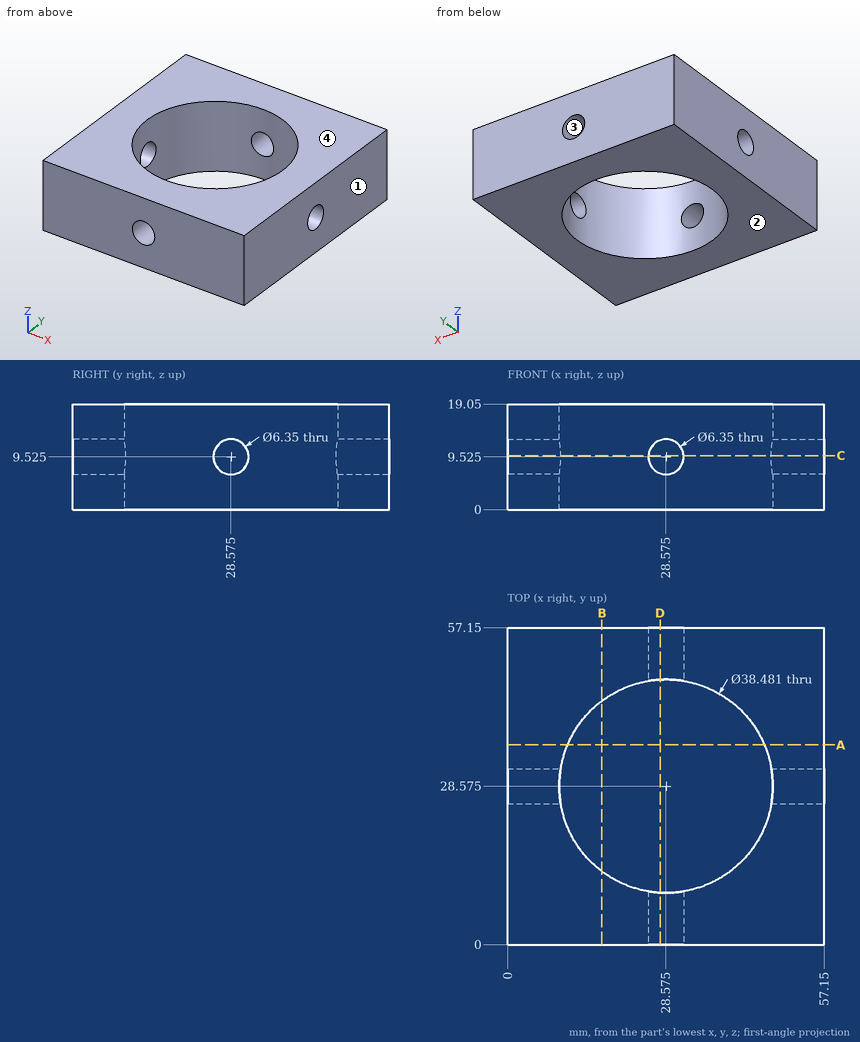
Could you check a few things on this drawing? It's one solid part, dimensions in mm from its lowest x, y, z. Give positions to 0.01 mm unless a question says otherwise; leave off trailing zeros. Loops run counter-clockwise (first coordinate to the right, second up) from the corner with the lowest first, then second, coordinate; pieces in that order, holes last. Notation, with made-up numbers: M -17.75,14 L 9.25,14 A26 cw 9.25,34 Z; hole C 63,35.5 d7. An arc over 180 degrees is marked long. Answer as a JSON object with one key per item and string values.
Q1. If we mould it in two halves opening along Z, with no side actions, what happens to the marked faces 1, 2, 3 and 4? For each: pulls with the +Z half, pulls with the -Z half, needs draft (parallel to the pull), parting line crosses it, or undercut.
Values found:
{"face 1": "needs draft", "face 2": "pulls with the -Z half", "face 3": "undercut", "face 4": "pulls with the +Z half"}
Q2. Suppose I cut it at D-D, the plane x = 27.5. List the corners of the cut face in (y, z) for me, plus the area to 3 significant figures.
Values found:
{"outline": "M 0,0 L 9.36,0 L 9.36,6.54 L 0,6.54 Z; M 0,12.51 L 9.36,12.51 L 9.36,19.05 L 0,19.05 Z; M 47.79,0 L 57.15,0 L 57.15,6.54 L 47.79,6.54 Z; M 47.79,12.51 L 57.15,12.51 L 57.15,19.05 L 47.79,19.05 Z", "area": "245 mm²"}
Q3. Suppose I cut it at C-C, the plane z = 9.75. State how many separate pieces and enclosed holes the cut face has, plus the area to 3 significant figures.
Values found:
{"separate pieces": "4", "enclosed holes": "0", "area": "1,860 mm²"}
Q4. If I drill on probe 1 along X at (y, z) = (5, 9.5); probe 2 along Y at (x, z) = (28, 16.5); probe 3 along X at (y, z) = (11, 15.25), over which ranges is the centre line in solid material (lowest first)? Write a range as [from, to].
Values found:
{"probe 1": "x = [0, 25.4], [31.75, 57.15]", "probe 2": "y = [0, 9.34], [47.81, 57.15]", "probe 3": "x = [0, 20.74], [36.41, 57.15]"}
Q5. For P1, Ø23, axis at x = 28.575, y = 28.575, coming from the +Z side, with a flat end and sliding along its axis, tell me the tip position at first contact or that it passes through.
Values found:
{"P1": "passes through"}
Q6. Suppose I cut it at B-B, the plane x = 17. List the corners of the cut face in (y, z) for me, plus the area to 3 significant figures.
Values found:
{"outline": "M 0,0 L 13.21,0 L 13.21,19.05 L 0,19.05 Z; M 43.94,0 L 57.15,0 L 57.15,19.05 L 43.94,19.05 Z", "area": "503 mm²"}
Q7. Suppose I cut it at A-A, the plane y = 36. List the corners of the cut face in (x, z) for me.
Values found:
{"outline": "M 0,0 L 10.82,0 L 10.82,19.05 L 0,19.05 Z; M 46.33,0 L 57.15,0 L 57.15,19.05 L 46.33,19.05 Z"}
